Design review of the part built by this model. Coordinates are the model's own, in mm. A direction names the side the tool comes from. Coordinates: 2 decimals unless noted, no trailing zeros. Order: outer loops, then holes, each group sorted by start corner. A loop starts at its lowest first (then second) coordinate and runs counter-clockwise, first axis right, second up. Notation, with made-up numbers: (84.5, -39.5) -> (132.5, -39.5) arc R18 cw to (132.5, -7.5) -> close; hole circle Ø2 at (-23.75, 46.25). An arc over 180 degrees is marked (long way). Use a Markdown table: item, result. Add a question column.
Q1. Insertion check: pin 1 (0.8 mm diameter, centred on x = -9, z = 76.5, fed in from +Y); pin 2 (3.5 mm diameter, centred on x = -0.5, z = 67.5, fed in from +Y); pin 3 (0.5 mm diameter, centred on y = 9, z = 120, fed in from -X). Each pin has a flat end and moves straight along its axis. Give the tip position at first contact, or say it passes through.
Q2. Add section A-A (x = 0.25). State the section outline as (y, z) points, then the cut area to 3 significant figures.
Q3. Machinability: for faces 4 (the face through (0, -3.65, 99)), 5 (the face through (6, 10, 99)), 6 (the face through (3.65, 0, 99)), which of the approach directions +Z, -Z, +X, -X, +Y, -Y give a long, thin tool a straight path to every point of the face, cutting with its end or side? Answer none if there is none.
Q4. Wall thickness on probe 1 along Y at (x, z) = (-3, 105); probe 2 along Y at (x, z) = (-3.25, 98): over which ranges is each line inside the solid? List them lowest first.
Q5. The part is to be moulded in two halves that separate along Y. For faces 1 (the face through (0, 0, 0)), 2 (the face through (-5, 10, 99)), 3 (the face through (-3.65, 0, 99)), say which applies: pulls with the +Y half, pulls with the -Y half, needs draft (parallel to the pull), parting line crosses it, or undercut.
from build123d import *

# Parameters (mm, degrees)
AUFSATZ_LINEAR_AUSTRAGEN1_DEPTH = 200
VERRUNDUNG1_R                   = 2
VERRUNDUNG2_R                   = 0.5


with BuildPart() as part:
    # Skizze1 → Aufsatz-Linear austragen1 (new body)
    with BuildSketch(Plane.XY):
        Polygon((-10, 2.5), (-8, 2.5), (-8, 6.85), (-3.65, 2.5), (-3.65, -2.5), (-8, -6.85), (-8, -2.5), (-10, -2.5), (-10, -10), (-2.5, -10), (-2.5, -8), (-6.85, -8), (-2.5, -3.65), (2.5, -3.65), (6.85, -8), (2.5, -8), (2.5, -10), (10, -10), (10, -2.5), (8, -2.5), (8, -6.85), (3.65, -2.5), (3.65, 2.5), (8, 6.85), (8, 2.5), (10, 2.5), (10, 10), (2.5, 10), (2.5, 8), (6.85, 8), (2.5, 3.65), (-2.5, 3.65), (-6.85, 8), (-2.5, 8), (-2.5, 10), (-10, 10), align=None)
    extrude(amount=AUFSATZ_LINEAR_AUSTRAGEN1_DEPTH)

    # Verrundung1
    verrundung1_edges = [part.edges().sort_by_distance(p)[0] for p in [
        (-10, 10, 100),
        (-10, -10, 100),
        (10, -10, 100),
        (10, 10, 100),
    ]]
    fillet(verrundung1_edges, radius=VERRUNDUNG1_R)

    # Verrundung2
    verrundung2_edges = [part.edges().sort_by_distance(p)[0] for p in [
        (-2.5, 10, 100),
        (-10, 2.5, 100),
        (-8, 2.5, 100),
        (-3.65, 2.5, 100),
        (-3.65, -2.5, 100),
        (-8, -2.5, 100),
        (-10, -2.5, 100),
        (-2.5, -10, 100),
        (-2.5, -8, 100),
        (-2.5, -3.65, 100),
        (2.5, -3.65, 100),
        (2.5, -8, 100),
        (2.5, -10, 100),
        (10, -2.5, 100),
        (8, -2.5, 100),
        (3.65, -2.5, 100),
        (3.65, 2.5, 100),
        (8, 2.5, 100),
        (10, 2.5, 100),
        (2.5, 10, 100),
        (2.5, 8, 100),
        (2.5, 3.65, 100),
        (-2.5, 3.65, 100),
        (-2.5, 8, 100),
    ]]
    fillet(verrundung2_edges, radius=VERRUNDUNG2_R)


solid = part.part
Established:
| question | item | result |
|---|---|---|
| 1 | pin 1 | y = 9.91 |
| 1 | pin 2 | y = 3.65 |
| 1 | pin 3 | x = -9.85 |
| 2 | outline | (-3.65, 0) -> (3.65, 0) -> (3.65, 200) -> (-3.65, 200) -> close |
| 2 | area | 1,460 mm^2 |
| 3 | face 4 | +Z, -Z, -Y |
| 3 | face 5 | +Z, -Z, +X, -X, +Y |
| 3 | face 6 | +Z, -Z, +X |
| 4 | probe 1 | -10 to -8, -4.15 to 4.15, 8 to 10 |
| 4 | probe 2 | -10 to -8, -4.4 to 4.4, 8 to 10 |
| 5 | face 1 | needs draft |
| 5 | face 2 | pulls with the +Y half |
| 5 | face 3 | undercut |
